```python
from build123d import *

# Parameters (mm, degrees)
BOSS_EXTRUDE1_DEPTH     = 6.35
CUT_EXTRUDE8_DEPTH      = 226.268216746
CUT_EXTRUDE8_DEPTH_BACK = 226.268216746
SKETCH35_R              = 2.38125
SKETCH36_W              = 12.7
SKETCH36_H              = 152.4
CUT_EXTRUDE9_DEPTH      = 226.268216746
SKETCH37_W              = 38.1
SKETCH37_H              = 101.6
CUT_EXTRUDE10_DEPTH     = 226.268216746


with BuildPart() as part:
    # Sketch1 → Boss-Extrude1 (new body)
    with BuildSketch(Plane(origin=(0, 0, 0), x_dir=(1, 0, 0), z_dir=(0, 1, 0))):
        Polygon((-177.8, -138.176), (-76.2, -138.176), (-76.2, -128.651), (76.2, -128.651), (76.2, -138.176), (177.8, -138.176), (177.8, -83.439), (168.275, -83.439), (168.275, -7.239), (177.8, -7.239), (177.8, 47.498), (-177.8, 47.498), (-177.8, -7.239), (-168.275, -7.239), (-168.275, -83.439), (-177.8, -83.439), align=None)
    extrude(amount=BOSS_EXTRUDE1_DEPTH)

    # Sketch35 → Cut-Extrude8 (cut, two sides: drawn at the far end of the back side and taken through both)
    with BuildSketch(Plane(origin=(0, 0, 0), x_dir=(-1, 0, 0), z_dir=(0, -1, 0)).offset(-CUT_EXTRUDE8_DEPTH_BACK)):
        with Locations(Location((-173.0375, 14.986, 0), (0, 0, 90))):
            Circle(SKETCH35_R)
        with Locations(Location((-173.0375, -108.839, 0), (0, 0, 90))):
            Circle(SKETCH35_R)
        with Locations(Location((-101.6, -133.4135, 0), (0, 0, 90))):
            Circle(SKETCH35_R)
        with Locations(Location((-127, -133.4135, 0), (0, 0, 90))):
            Circle(SKETCH35_R)
        with Locations(Location((-152.4, -133.4135, 0), (0, 0, 90))):
            Circle(SKETCH35_R)
        with Locations(Location((101.6, -133.4135, 0), (0, 0, 270))):
            Circle(SKETCH35_R)
        with Locations(Location((127, -133.4135, 0), (0, 0, 270))):
            Circle(SKETCH35_R)
        with Locations(Location((152.4, -133.4135, 0), (0, 0, 270))):
            Circle(SKETCH35_R)
        with Locations(Location((173.0375, -108.839, 0), (0, 0, 270))):
            Circle(SKETCH35_R)
        with Locations(Location((173.0375, 14.986, 0), (0, 0, 270))):
            Circle(SKETCH35_R)
    extrude(amount=CUT_EXTRUDE8_DEPTH + CUT_EXTRUDE8_DEPTH_BACK, mode=Mode.SUBTRACT)

    # Sketch36 → Cut-Extrude9 (cut, through all)
    with BuildSketch(Plane.XZ):
        with Locations((-28.575, -3.302)):
            Rectangle(SKETCH36_W, SKETCH36_H)
        with Locations((28.575, -3.302)):
            Rectangle(SKETCH36_W, SKETCH36_H)
    extrude(amount=-CUT_EXTRUDE9_DEPTH, mode=Mode.SUBTRACT)

    # Sketch37 → Cut-Extrude10 (cut, through all)
    with BuildSketch(Plane.XZ):
        with Locations((-139.7, 42.799)):
            Rectangle(SKETCH37_W, SKETCH37_H)
        with Locations((139.7, 42.799)):
            Rectangle(SKETCH37_W, SKETCH37_H)
    extrude(amount=-CUT_EXTRUDE10_DEPTH, mode=Mode.SUBTRACT)


solid = part.part
```
Model file for the job. Use its own axes, mm. A direction names the side the tool comes from. Coordinates: 2 decimals unless noted, no trailing zeros. Loops run counter-clockwise (first coordinate to the right, second up) from the corner with the lowest first, then second, coordinate; pieces in that order, holes last. Notation, with made-up numbers: M 29.25,-9.5 L 75.25,-9.5 A26 cw 75.25,24.5 Z; hole C 78.5,58 d5. An arc over 180 degrees is marked long. Use CSV: the item, a comma, the result in double quotes. Start each with the question number.
1. Flat gauge pins, fed straight in: pin 1 (4 mm diameter, centred on x = 101.6, z = 133.41, fed in from -Y); pin 2 (1.5 mm diameter, centred on x = -38.5, z = 45, fed in from -Y); pin 3 (2 mm diameter, centred on y = 2, z = 29, fed in from -X) (3 decimals); pin 4 (1.5 mm diameter, centred on x = 11, y = 1, fed in from +Z). Where does each tip first touch, or does it go through?
2. Two-plate mould, pull along Z, no slides. Class faces 1 (the flat face through (-105, 3, -47.498)), 2 (the flat face through (-140, 3, 93.599)), 3 (the flat face through (-2, 0, 44)): pulls with the +Z half, pulls with the -Z half, needs draft (parallel to the pull), parting line crosses it, or undercut.
3. Probe probe 1 along X at (y, z) = (4.25, 17) (3 decimals); probe 2 along X at (y, z) = (6.25, 73) (3 decimals); probe 3 along X at (y, z) = (1, -27.5) (3 decimals). List the from-to ranges inside material, lowest first. Write a range as [from, to].
4. Band-saw the part on C-C, the plane y = 1. Give the number of separate pieces and of enclosed holes in the cut face, then the cut area to 3 significant figures.
5. Tool access for faces 4 (the flat face through (173, 3, 7.239)), 5 (the flat face through (139, 3, -8.001)), 6 (the flat face through (-34.925, 3, 12)), 7 (the flat face through (-173, 3, 7.239)), 8 (the flat face through (177.8, 3, -20)): list every direction of +Z, -Z, +X, -X, +Y, -Y with a clear straight run to the whole face (end or side of a thin tool).
6. Band-saw the part on A-A, the plane z = 59.5. List the corners of the cut face in (x, y) (3 decimals).
7. Band-saw the part on D-D, the plane x = 61.5. List the corners of the cut face in (y, z).
8. Band-saw the part on B-B, the plane x = -28. List the corners of the cut face in (y, z), then the cut area to 3 significant figures.
Entries:
1,pin 1,"passes through"
1,pin 2,"stops at y = 0"
1,pin 3,"stops at x = -168.275"
1,pin 4,"stops at z = 128.65"
2,face 1,"pulls with the -Z half"
2,face 2,"undercut"
2,face 3,"needs draft"
3,probe 1,"x = [-168.275, -158.75], [-120.65, -34.925], [-22.225, 22.225], [34.925, 120.65], [158.75, 168.275]"
3,probe 2,"x = [-168.275, -158.75], [-120.65, 120.65], [158.75, 168.275]"
3,probe 3,"x = [-177.8, -34.925], [-22.225, 22.225], [34.925, 177.8]"
4,separate pieces,"1"
4,enclosed holes,"12"
4,area,"52,100 mm2"
5,face 4,"+X, +Y, -Y"
5,face 5,"+Y, -Y"
5,face 6,"-Z, +Y, -Y"
5,face 7,"-X, +Y, -Y"
5,face 8,"+Z, -Z, +X, +Y, -Y"
6,outline,"M -168.275,0 L -158.75,0 L -158.75,6.35 L -168.275,6.35 Z; M -120.65,0 L -34.925,0 L -34.925,6.35 L -120.65,6.35 Z; M -22.225,0 L 22.225,0 L 22.225,6.35 L -22.225,6.35 Z; M 34.925,0 L 120.65,0 L 120.65,6.35 L 34.925,6.35 Z; M 158.75,0 L 168.275,0 L 168.275,6.35 L 158.75,6.35 Z"
7,outline,"M 0,-47.5 L 6.35,-47.5 L 6.35,128.65 L 0,128.65 Z"
8,outline,"M 0,72.9 L 6.35,72.9 L 6.35,128.65 L 0,128.65 Z"
8,area,"354 mm2"
